from build123d import *

# Parameters (mm, degrees)
CUT_EXTRUDE_1_DEPTH = 2.5


with BuildPart() as part:
    # Эскиз1 → Повернуть1 (revolve)
    with BuildSketch(Plane.XY):
        Polygon((0, 0), (3, 0), (3, 8.4), (6, 11.4), (6, 12), (0, 12), align=None)
    revolve(axis=Axis((0, 68.644575989, 0), (0, -1, 0)))

    # Эскиз2 → Вырез-Вытянуть1 (cut)
    with BuildSketch(Plane(origin=(0, 12, 0), x_dir=(1, 0, 0), z_dir=(0, 1, 0))):
        Polygon((1.755265403, -2.986476748), (3.463997433, 0.026866056), (1.708732029, 3.013342804), (-1.755265403, 2.986476748), (-3.463997433, -0.026866056), (-1.708732029, -3.013342804), align=None)
    extrude(amount=-CUT_EXTRUDE_1_DEPTH, mode=Mode.SUBTRACT)


solid = part.part
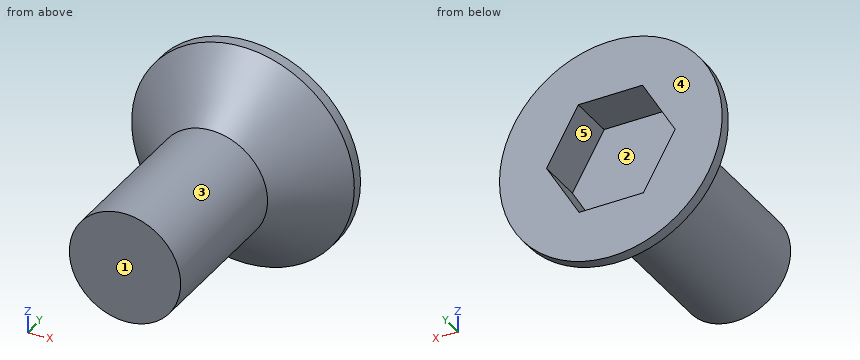
Verification items for the finished model (mm, model axes). Face numbers are marked on the shaded views. A direction names the side the tool comes from. Coordinates: 2 decimals unless noted, no trailing zeros. Order: outer loops, then holes, each group sorted by start corner. A loop starts at its lowest first (then second) coordinate and runs counter-clockwise, first axis right, second up.
1. Release check for a two-part mould opening along Z. For the marked faces 3, 4 and 5 record: +Z half, -Z half, draft (parallel to the pull), parting line (faces both ways), or undercut.
Results found:
face 3: parting line
face 4: draft
face 5: undercut
2. Sectioned sample at B-B, the plane x = 0. Record the cut outline in (y, z), and give its area (3 significant figures).
Results found:
outline: (0, -3) - (8.4, -3) - (11.4, -6) - (12, -6) - (12, -3) - (9.5, -3) - (9.5, 3) - (12, 3) - (12, 6) - (11.4, 6) - (8.4, 3) - (0, 3) - close
area: 69.6 mm2
3. Set-up check for the marked faces 1 and 2: record each of +Z, -Z, +X, -X, +Y, -Y from which the full face is reachable in a straight line by a thin tool's end or side.
Results found:
face 1: +Z, -Z, +X, -X, -Y
face 2: +Y
4. Scan lines: line 1 (Y direction, x = 1.25, z = -2.25); line 2 (X direction, y = 6.25, z = -0.25); line 3 (Y direction, x = -2.5, z = -5.25). Record each from-to range of solid material in increasing order.
Results found:
line 1: y = 0 to 9.5
line 2: x = -2.99 to 2.99
line 3: y = 11.21 to 12
5. Sectioned sample at C-C, the plane y = 2. Record the cut outline in (x, z), and give its area (3 significant figures).
Results found:
outline: circle Ø6 at (0, 0)
area: 28.3 mm2
6. Go/stop test with flat-tipped pins: pin 1 Ø2 at (x, z) = (-0.5, 4.5) entering from -Y; pin 2 Ø1 at (x, y) = (-3, 7.5) entering from +Z; pin 3 Ø3 at (x, y) = (3.5, 4) entering from -Z. Record where each tip stops, or that it passes through.
Results found:
pin 1: stops at y = 8.93
pin 2: stops at z = 1.66
pin 3: stops at z = -2.24
7. Sectioned sample at A-A, the plane y = 11. Record the cut outline in (x, z), and give its area (3 significant figures).
Results found:
outline: circle Ø11.2 at (0, 0); hole (-3.46, 0.03) - (-1.76, -2.99) - (1.71, -3.01) - (3.46, -0.03) - (1.76, 2.99) - (-1.71, 3.01) - close
area: 67.3 mm2
